Can you work these out from the model? Positions are in its coordinate system, mm. Give positions to 0.01 mm unless a question says otherwise; leave off trailing zeros. Order: outer loops, then holes, each group sorted by start corner. A loop starts at its lowest first (then second) coordinate and runs counter-clockwise, first axis right, second up.
Item 1: I want a section at B-B, the plane x = -4. Write out the boundary of the cut face in (y, z) (3 decimals).
Item 2: I want a section at C-C, the plane z = 6.5. Count the separate pieces of the cut face and the enclosed holes in it, then the cut area to 3 significant figures.
Item 3: If I drill on line 1 along X through (y, z) = (1.6, 11.75); line 2 along Y through (x, z) = (7.5, 13) (1 decimal); line 3 along X through (y, z) = (0.65, 16), over which ranges is the centre line in solid material (lowest first)?
Item 4: I'm going to push a flat-ended pin straight in: pin 1 Ø1.5 at (x, y) = (31.25, 1.59) entering from +Z. Where does the tip first touch, or does it pass through?
Item 5: I want a section at A-A, the plane z = 0. Write out the boundary of the cut face in (x, y) (3 decimals).
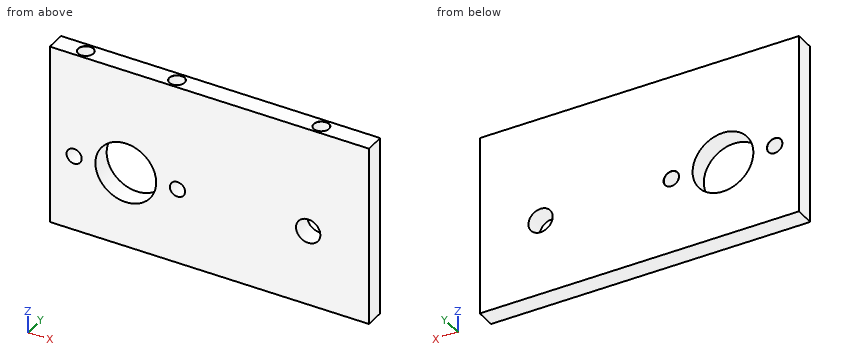
```python
from build123d import *

# Parameters (mm, degrees)
BOSS_EXTRUDE1_DEPTH                   = 3.175
TAP_DRILL_FOR_M3X0_5_TAP1_D           = 2.5
TAP_DRILL_FOR_M3X0_5_TAP1_CSINK_D     = 2.55
TAP_DRILL_FOR_M3X0_5_TAP1_CSINK_ANGLE = 90
CUT_EXTRUDE1_REACH                    = 23.61
SKETCH8_R                             = 5
SKETCH9_W                             = 27.5
SKETCH9_H                             = 29.84
SKETCH9_R                             = 2
BOSS_EXTRUDE2_DEPTH                   = 3.175
TAP_DRILL_FOR_M3X0_5_TAP2_D           = 2.5
TAP_DRILL_FOR_M3X0_5_TAP2_DEPTH       = 12
TAP_DRILL_FOR_M3X0_5_TAP2_CSINK_D     = 2.55
TAP_DRILL_FOR_M3X0_5_TAP2_CSINK_ANGLE = 90
TAP_DRILL_FOR_M3X0_5_TAP2_TIP         = 0.751075774


with BuildPart() as part:
    # Sketch1 → Boss-Extrude1 (new body)
    with BuildSketch(Plane(origin=(0, 0, 0), x_dir=(1, 0, 0), z_dir=(0, 1, 0))):
        Polygon((-12.5, -12.5), (-12.5, -17.34), (12.5, -17.34), (12.5, -12.5), (12.5, 12.5), (-12.5, 12.5), align=None)
    extrude(amount=BOSS_EXTRUDE1_DEPTH)

    # Tap Drill for M3x0.5 Tap1 (through all)
    with Locations(Plane(origin=(0, 3.175, 0), x_dir=(1, 0, 0), z_dir=(0, 1, 0))):
        with Locations((-8.5, 0), (8.5, 0)):
            CounterSinkHole(TAP_DRILL_FOR_M3X0_5_TAP1_D / 2, TAP_DRILL_FOR_M3X0_5_TAP1_CSINK_D / 2, counter_sink_angle=TAP_DRILL_FOR_M3X0_5_TAP1_CSINK_ANGLE)

    # Sketch8 → Cut-Extrude1 (cut, up to next)
    with BuildSketch(Plane(origin=(0, 3.175, 0), x_dir=(1, 0, 0), z_dir=(0, 1, 0)), mode=Mode.PRIVATE) as cut_extrude1_sk1:
        with Locations(Location((0, 0, 0), (0, 0, 270))):
            Circle(SKETCH8_R)
    cut_extrude1_tool1 = extrude(cut_extrude1_sk1.sketch, amount=-CUT_EXTRUDE1_REACH, mode=Mode.PRIVATE) & part.part
    add(cut_extrude1_tool1.solids().sort_by_distance((0, 3.175, 0))[0], mode=Mode.SUBTRACT)

    # Sketch9 → Boss-Extrude2 (add)
    with BuildSketch(Plane(origin=(0, 3.175, 0), x_dir=(1, 0, 0), z_dir=(0, 1, 0))):
        with Locations((26.25, -2.42)):
            Rectangle(SKETCH9_W, SKETCH9_H)
        with Locations(Location((30, 0, 0), (0, 0, 270))):
            Circle(SKETCH9_R, mode=Mode.SUBTRACT)
    extrude(amount=-BOSS_EXTRUDE2_DEPTH)

    # Tap Drill for M3x0.5 Tap2
    with Locations(Plane.XY.offset(17.34)):
        with Locations((-7.5, 1.5875), (7.5, 1.5875), (31.25, 1.5875)):
            CounterSinkHole(TAP_DRILL_FOR_M3X0_5_TAP2_D / 2, TAP_DRILL_FOR_M3X0_5_TAP2_CSINK_D / 2, depth=TAP_DRILL_FOR_M3X0_5_TAP2_DEPTH, counter_sink_angle=TAP_DRILL_FOR_M3X0_5_TAP2_CSINK_ANGLE)
            with Locations((0, 0, -(TAP_DRILL_FOR_M3X0_5_TAP2_DEPTH + TAP_DRILL_FOR_M3X0_5_TAP2_TIP / 2))):  # 118° drill point
                Cone(0, TAP_DRILL_FOR_M3X0_5_TAP2_D / 2, TAP_DRILL_FOR_M3X0_5_TAP2_TIP, mode=Mode.SUBTRACT)


solid = part.part
```
Results list:
1. outline: (0, -12.5) - (3.175, -12.5) - (3.175, -3) - (0, -3) - close; (0, 3) - (3.175, 3) - (3.175, 17.34) - (0, 17.34) - close
2. separate pieces: 1
2. enclosed holes: 3
2. area: 152 mm2
3. line 1: x = -12.5 to -8.75, -6.25 to 6.25, 8.75 to 30, 32.5 to 40
3. line 2: y = 0 to 0.3, 2.8 to 3.2
3. line 3: x = -12.5 to -8.33, -6.67 to 6.67, 8.33 to 30.42, 32.08 to 40
4. pin 1: stops at z = 5.04
5. outline: (-12.5, 0) - (-9.75, 0) - (-9.75, 3.15) - (-9.775, 3.175) - (-12.5, 3.175) - close; (-7.25, 0) - (-5, 0) - (-5, 3.175) - (-7.225, 3.175) - (-7.25, 3.15) - close; (5, 0) - (7.25, 0) - (7.25, 3.15) - (7.225, 3.175) - (5, 3.175) - close; (9.75, 0) - (28, 0) - (28, 3.175) - (9.775, 3.175) - (9.75, 3.15) - close; (32, 0) - (40, 0) - (40, 3.175) - (32, 3.175) - close
